from build123d import *

# Parameters (mm, degrees)
SKETCH1_W           = 42
SKETCH1_H           = 5.9
SKETCH1_W_2         = 39.9
SKETCH1_H_2         = 3.5
BOSS_EXTRUDE1_DEPTH = 32.25
FILLET2_R           = 3
SKETCH2_W           = 51.5
SKETCH2_H           = 13.6
SKETCH2_W_2         = 39.9
SKETCH2_H_2         = 3.5
BOSS_EXTRUDE2_DEPTH = 5.8
SKETCH3_W           = 51.5
SKETCH3_H           = 13.6
SKETCH3_W_2         = 39.9
SKETCH3_H_2         = 3.5
BOSS_EXTRUDE3_DEPTH = 5.8
SKETCH4_R           = 1.6
CUT_EXTRUDE1_DEPTH  = 62.792596644
BOSS_EXTRUDE4_DEPTH = 13.6
CUT_EXTRUDE4_DEPTH  = 4
SKETCH15_W          = 39.9
SKETCH15_H          = 3.5
CUT_EXTRUDE5_DEPTH  = 74.483654645
SKETCH17_R          = 2
CUT_EXTRUDE6_DEPTH  = 74.483654645


with BuildPart() as part:
    # Sketch1 → Boss-Extrude1 (new body)
    with BuildSketch(Plane(origin=(0, 0, 0), x_dir=(0, 0, -1), z_dir=(1, 0, 0))):
        with Locations((21, 2.95)):
            Rectangle(SKETCH1_W, SKETCH1_H)
        with Locations((21, 2.95)):
            Rectangle(SKETCH1_W_2, SKETCH1_H_2, mode=Mode.SUBTRACT)
    extrude(amount=BOSS_EXTRUDE1_DEPTH)

    # Fillet2
    # the kernel refuses this fillet: 3 mm, written as the material it takes off along each edge
    with BuildSketch(Plane(origin=(-7.5, 0, -42), x_dir=(0, 0, 1), z_dir=(1, 0, 0)), Plane(origin=(-7.5, 5.9, 0), x_dir=(0, 0, -1), z_dir=(1, 0, 0)), Plane(origin=(-7.5, 5.9, -42), x_dir=(0, -1, 0), z_dir=(1, 0, 0))) as fillet2_piece_1:
        with BuildLine():
            CenterArc((FILLET2_R, -FILLET2_R), FILLET2_R, 90, 90)
            Line((0, -FILLET2_R), (0, 0))
            Line((0, 0), (FILLET2_R, 0))
        make_face()
    extrude(amount=47.25, mode=Mode.SUBTRACT)
    with BuildSketch(Plane(origin=(-7.5, 0, 0), x_dir=(0, 0, -1), z_dir=(1, 0, 0))) as fillet2_piece_2:
        with BuildLine():
            CenterArc((FILLET2_R, FILLET2_R), FILLET2_R, 180, 90)
            Line((0, FILLET2_R), (0, 0))
            Line((0, 0), (FILLET2_R, 0))
        make_face()
    extrude(amount=47.25, mode=Mode.SUBTRACT)

    # Sketch2 → Boss-Extrude2 (add)
    with BuildSketch(Plane(origin=(32.25, 0, 0), x_dir=(0, 0, -1), z_dir=(1, 0, 0))):
        with Locations((21, 2.95)):
            Rectangle(SKETCH2_W, SKETCH2_H)
        with Locations((21, 2.95)):
            Rectangle(SKETCH2_W_2, SKETCH2_H_2, mode=Mode.SUBTRACT)
    extrude(amount=BOSS_EXTRUDE2_DEPTH)

    # Sketch3 → Boss-Extrude3 (add)
    with BuildSketch(Plane.ZY):
        with Locations((-21, 2.95)):
            Rectangle(SKETCH3_W, SKETCH3_H)
        with Locations((-21, 2.95)):
            Rectangle(SKETCH3_W_2, SKETCH3_H_2, mode=Mode.SUBTRACT)
    extrude(amount=BOSS_EXTRUDE3_DEPTH)

    # Sketch4 → Cut-Extrude1 (cut, through all)
    with BuildSketch(Plane(origin=(0, 9.75, 0), x_dir=(1, 0, 0), z_dir=(0, 1, 0))):
        with Locations(Location((-2.9, 43.85, 0), (0, 0, 270))):
            Circle(SKETCH4_R)
        with Locations(Location((35.15, 43.85, 0), (0, 0, 270))):
            Circle(SKETCH4_R)
        with Locations(Location((-2.9, -1.85, 0), (0, 0, 270))):
            Circle(SKETCH4_R)
        with Locations(Location((35.15, -1.85, 0), (0, 0, 270))):
            Circle(SKETCH4_R)
    extrude(amount=-CUT_EXTRUDE1_DEPTH, mode=Mode.SUBTRACT)

    # Sketch8 → Boss-Extrude4 (add)
    with BuildSketch(Plane(origin=(0, 9.75, 0), x_dir=(1, 0, 0), z_dir=(0, 1, 0))):
        with BuildLine():
            ThreePointArc((46.05, 17), (50.05, 21), (46.05, 25))
            Line((46.05, 25), (46.05, 41.999583304))
            Line((46.05, 41.999583304), (38.05, 41.999583304))
            Line((38.05, 41.999583304), (38.05, 0.000416696))
            Line((38.05, 0.000416696), (46.05, 0.000416696))
            Line((46.05, 0.000416696), (46.05, 17))
        make_face()
    extrude(amount=-BOSS_EXTRUDE4_DEPTH)

    # Sketch13 → CSK for M2 Flat Head Machine Screw1 (revolve, cut)
    with BuildSketch(Plane(origin=(46.05, 9.75, -21), x_dir=(0, 0, 1), z_dir=(1, 0, 0))):
        Polygon((0, 0), (0, 13.6), (1, 13.6), (1, 3.75), (2, 2.75), (2, 0), align=None)
    revolve(axis=Axis((46.05, 16.1, -21), (0, -1, 0)), mode=Mode.SUBTRACT)

    # Sketch14 → Cut-Extrude4 (cut)
    with BuildSketch(Plane.XZ.offset(3.85)):
        Polygon((43.671623782, -20.5274256), (44.451550455, -22.823447025), (46.829926673, -23.296021425), (48.428376218, -21.4725744), (47.648449545, -19.176552975), (45.270073327, -18.703978575), align=None)
    extrude(amount=-CUT_EXTRUDE4_DEPTH, mode=Mode.SUBTRACT)

    # Sketch15 → Cut-Extrude5 (cut, through all)
    with BuildSketch(Plane.ZY.offset(5.8)):
        with Locations((-21, 2.95)):
            Rectangle(SKETCH15_W, SKETCH15_H)
    extrude(amount=-CUT_EXTRUDE5_DEPTH, mode=Mode.SUBTRACT)

    # Sketch17 → Cut-Extrude6 (cut, through all)
    with BuildSketch(Plane.ZY.offset(5.8)):
        with Locations((-21, 2.95)):
            Circle(SKETCH17_R)
    extrude(amount=-CUT_EXTRUDE6_DEPTH, mode=Mode.SUBTRACT)


solid = part.part
Read the model definition and answer for the solid it produces. Units are mm, in the model's axes. A direction names the side the tool comes from. Round coordinates to 2 decimals unless told otherwise and drop trailing zeros. Order: outer loops, then holes, each group sorted by start corner. A loop starts at its lowest first (then second) coordinate and runs counter-clockwise, first axis right, second up.
1) Flat-ended cylindrical pins translate along their axes: pin 1 (21 mm diameter, centred on x = 18, z = -6.5, fed in from -Y); pin 2 (4 mm diameter, centred on x = 42.5, y = 3.5, fed in from +Z); pin 3 (1.4 mm diameter, centred on y = 2.5, z = 1.5, fed in from +X); pin 4 (1.8 mm diameter, centred on x = 46.05, z = -21, fed in from +Y). Find the tip coordinate at first contact, or state that the pin passes through.
2) The mould has two halves that part along Z. Classify faces 1 (the face through (-5.8, 6, -21)), 2 (the face through (50.05, 7.26, -20.91)), 3 (the face through (44.056, -1.878, -21.659)), 4 (the face through (-4.32, 3.05, 2.59)): released by +Z, released by -Z, zero draft, split by the parting line, or undercut.
3) The part is cut by section A-A on x = 35.15. Write down the section's boundary in (y, z).
4) The part is cut by section B-B on z = -11. Write down the section's boundary in (x, y).
5) For faces 5 (the face through (38.05, 3, 2)), 6 (the face through (46, 5, -20)), 7 (the face through (44.698, 8.394, -22.474)), 8 (the face through (44.482, -1.878, -19.603)), 9 (the face through (48.57, 0.95, -21.01)), determine the directions among +Z, -Z, +X, -X, +Y, -Y from which every point of the face is accessible in a straight line to the end or side of a thin tool.
6) The part is cut by section D-D on x = 25. Write down the section's boundary in (y, z).
7) The part is cut by section C-C on y = 2.25. Write down the section's boundary in (x, z), plus the area to 3 significant figures.
8) Straight lines are drawn through the part: L1, parallel to X at y = 6.25, z = 1.85; L2, parallel to X at y = 9.05, z = -21; L3, parallel to X at y = 5.05, z = -21. For each, find the intervals that lie inside material, in ascending order.
Resolved:
1. pin 1: stops at y = 0
1. pin 2: stops at z = 0
1. pin 3: stops at x = 38.05
1. pin 4: passes through
2. face 1: zero draft
2. face 2: split by the parting line
2. face 3: undercut
2. face 4: undercut
3. outline: (-3.85, -46.75) - (9.75, -46.75) - (9.75, -45.45) - (-3.85, -45.45) - close; (-3.85, -42.25) - (9.75, -42.25) - (9.75, 0.25) - (-3.85, 0.25) - close; (-3.85, 3.45) - (9.75, 3.45) - (9.75, 4.75) - (-3.85, 4.75) - close; hole (1.2, -40.95) - (4.7, -40.95) - (4.7, -21.97) arc R2 ccw to (4.7, -20.03) - (4.7, -1.05) - (1.2, -1.05) - (1.2, -20.03) arc R2 ccw to (1.2, -21.97) - close
4. outline: (-5.8, -3.85) - (0, -3.85) - (0, 0) - (32.25, 0) - (32.25, -3.85) - (46.05, -3.85) - (46.05, 1.2) - (-5.8, 1.2) - close; (-5.8, 4.7) - (46.05, 4.7) - (46.05, 9.75) - (32.25, 9.75) - (32.25, 5.9) - (0, 5.9) - (0, 9.75) - (-5.8, 9.75) - close
5. face 5: +Z, +X, +Y, -Y
5. face 6: +Y, -Y
5. face 7: +Y
5. face 8: -Y
5. face 9: +X, -X
6. outline: (0, -39) arc R3 ccw to (2.95, -42) arc R3 ccw to (5.9, -39) - (5.9, -3) arc R3 ccw to (2.95, 0) arc R3 ccw to (0, -3) - close; hole (1.2, -40.95) - (4.7, -40.95) - (4.7, -21.97) arc R2 ccw to (4.7, -20.03) - (4.7, -1.05) - (1.2, -1.05) - (1.2, -20.03) arc R2 ccw to (1.2, -21.97) - close
7. outline: (-5.8, -46.75) - (0, -46.75) - (0, -41.9) - (32.25, -41.9) - (32.25, -46.75) - (38.05, -46.75) - (38.05, -42) - (46.05, -42) - (46.05, -40.95) - (-5.8, -40.95) - close; (-5.8, -1.05) - (46.05, -1.05) - (46.05, 0) - (38.05, 0) - (38.05, 4.75) - (32.25, 4.75) - (32.25, -0.1) - (0, -0.1) - (0, 4.75) - (-5.8, 4.75) - close; hole circle Ø3.2 at (-2.9, -43.85); hole circle Ø3.2 at (-2.9, 1.85); hole circle Ø3.2 at (35.15, -43.85); hole circle Ø3.2 at (35.15, 1.85)
7. area: 181 mm2
8. L1: x = -5.8 to -4.5, -1.3 to 0, 32.25 to 33.55, 36.75 to 38.05
8. L2: x = -5.8 to 0, 32.25 to 44.05, 48.05 to 50.05
8. L3: x = -5.8 to 45.05, 47.05 to 50.05
